Geometry check sheet. Reference: drawing and pictorial views, mm from the part's lowest x, y, z. A direction names the side the tool comes from. Round coordinates to 2 decimals unless told otherwise and drop trailing zeros. Order: outer loops, then holes, each group sorted by start corner. A loop starts at its lowest first (then second) coordinate and runs counter-clockwise, first axis right, second up. Notation, with made-up numbers: (42, 7.25) -> (75, 7.25) arc R21 cw to (75, 36.25) -> close; hole circle Ø8 at (22.25, -33.75). An arc over 180 degrees is marked (long way). Put each result on its own line as item: value.
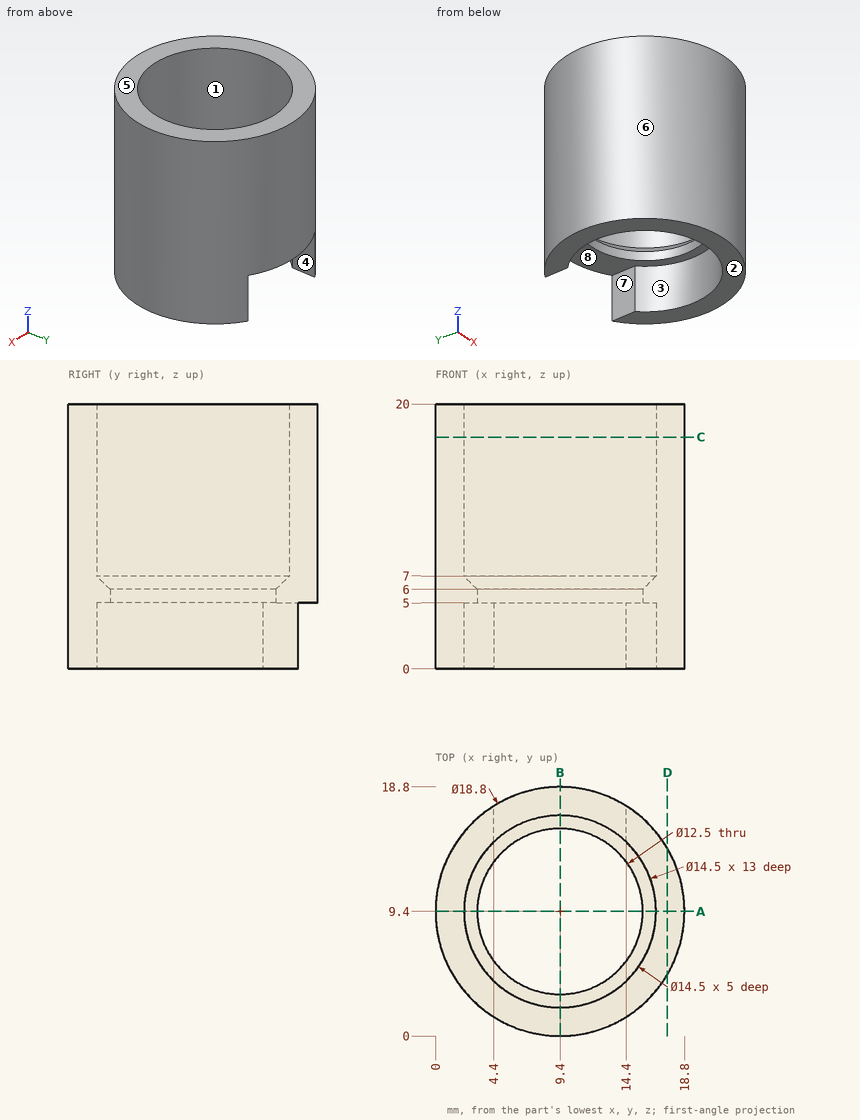
Item 1: Tool access check on the marked faces 1, 2, 3, 4 and 5. Record the directions out of +Z, -Z, +X, -X, +Y, -Y that give a thin tool (end or side, any length) a straight path to the whole face; none if there is none.
Geometry check:
face 1: +Z
face 2: -Z, +X, -X, +Y, -Y
face 3: -Z
face 4: -Z, +Y
face 5: +Z, +X, -X, +Y, -Y
Item 2: Sectioned sample at A-A, the plane y = 9.4. Record the boundary of the cut face in (x, z).
Geometry check:
outline: (0, 0) -> (2.15, 0) -> (2.15, 5) -> (3.15, 5) -> (3.15, 6) -> (2.15, 7) -> (2.15, 20) -> (0, 20) -> close; (15.65, 5) -> (16.65, 5) -> (16.65, 0) -> (18.8, 0) -> (18.8, 20) -> (16.65, 20) -> (16.65, 7) -> (15.65, 6) -> close
Item 3: Sectioned sample at B-B, the plane x = 9.4. Record the boundary of the cut face in (y, z).
Geometry check:
outline: (0, 0) -> (2.15, 0) -> (2.15, 5) -> (3.15, 5) -> (3.15, 6) -> (2.15, 7) -> (2.15, 20) -> (0, 20) -> close; (15.65, 5) -> (18.8, 5) -> (18.8, 20) -> (16.65, 20) -> (16.65, 7) -> (15.65, 6) -> close
Item 4: Release check for a two-part mould opening along Y. For the marked faces 6, 7 and 8 record: pulls with the +Y half, pulls with the -Y half, needs draft (parallel to the pull), parting line crosses it, or undercut.
Geometry check:
face 6: parting line crosses it
face 7: needs draft
face 8: undercut
Item 5: Sectioned sample at D-D, the plane x = 17.5. Record the boundary of the cut face in (y, z), then the cut area to 3 significant figures.
Geometry check:
outline: (4.63, 0) -> (14.17, 0) -> (14.17, 20) -> (4.63, 20) -> close
area: 191 mm2
Item 6: Depth check by flat-ended pin: pin 1 Ø6 at (y, z) = (4.5, 15) entering from -X; pin 2 Ø1 at (y, z) = (13, 10.5) entering from +X; pin 3 Ø1.4 at (y, z) = (16, 3.5) entering from +X; pin 4 Ø10 at (x, y) = (7, 3.5) entering from +Z. Enter the tip coordinate at first touch or a pass-through.
Geometry check:
pin 1: x = 0.19
pin 2: x = 18.27
pin 3: x = 16.72
pin 4: z = 20
Item 7: Material ranges on line 1 along Y through (x, z) = (9.4, 5.25); line 2 along Y through (x, z) = (9.4, 3.6); line 3 along Y through (x, z) = (4.75, 14.75), recorded low to high.
Geometry check:
line 1: 0 to 3.15, 15.65 to 18.8
line 2: 0 to 2.15
line 3: 1.23 to 3.84, 14.96 to 17.57
Item 8: Sectioned sample at C-C, the plane z = 17.5. Record the boundary of the cut face in (x, y), then the cut area to 3 significant figures.
Geometry check:
outline: circle Ø18.8 at (9.4, 9.4); hole circle Ø14.5 at (9.4, 9.4)
area: 112 mm2
